Could you check a few things on this model? Use its own coordinates, in mm. Face numbers are marked on the shaded views. A direction names the side the tool comes from. Coordinates: 2 decimals unless noted, no trailing zeros. Loops run counter-clockwise (first coordinate to the right, second up) from the corner with the lowest first, then second, coordinate; pieces in that order, holes last.
1) Imagine slicing it at B-B on x = -8. Please give me the cut outline in (y, z), plus the area to 3 significant figures.
2) For the marked faces 1, 2, 3, 4 and 5, which set-ups out of +Z, -Z, +X, -X, +Y, -Y let a thin tool reach every point of the face, with its end or its side?
3) Imagine slicing it at A-A on z = 24.25. Please give me the cut outline in (x, y).
4) If I drill on line 1 along Z through (x, y) = (-0.25, 13); line 2 along X through (y, z) = (12, -12); line 3 along X through (y, z) = (3.5, -3), over which ranges is the centre line in solid material (lowest first)?
5) Imagine slicing it at D-D on x = 10.25. Please give me the cut outline in (y, z).
6) Imagine slicing it at C-C on y = 19.5. Please give me the cut outline in (x, z).
7) Will these pins go through, and if not, where does the flat tip stop? P1, Ø12, axis at x = -7, z = 8, coming from the +Y side; P2, Ø4, axis at x = 8, z = -12.25, coming from the -Y side; P3, Ø6.5, axis at x = -1.5, z = 12, coming from the -Y side.
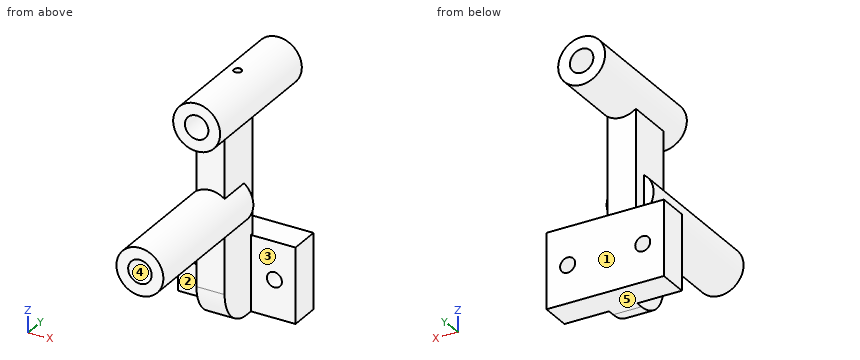
Autodesk Inventor part; units mm, degrees
ref_plane "Work Plane1" through (0, 0, 29.25) normal (0, 0, 1) x (1, 0, 0)
ref_plane "YZ Plane" through (0, 0, 0) normal (1, 0, 0) x (0, 1, 0)
ref_plane "XZ Plane" through (0, 0, 0) normal (0, 1, 0) x (-1, 0, 0)
sketch "Sketch1" plane through (0, 0, 0) normal (0, 1, 0) x (-1, 0, 0)
  line L0 (3, 20.25) -> (-3, 20.25)
  line L1 (-3, 20.25) -> (-3, -20.25)
  line L2 (-3, -20.25) -> (3, -20.25)
  line L3 (3, -20.25) -> (3, 20.25)
  line L4 (3, 20.25) -> (-3, -20.25) construction
  line L5 (-3, 20.25) -> (3, -20.25) construction
  point P0 (0, 0)
  dimension "d0" = 6
  dimension "d1" = 40.5
extrude "Extrusion1" add sketch "Sketch1" along normal blind 10
fillet "Fillet1" radius 8 1 edges at (0, 0, -20.25)
sketch "Sketch2" plane through (0, 10, 0) normal (0, 1, 0) x (1, 0, 0)
  line L0 (3, 20.25) -> (-3, 20.25) construction
  line L1 (0, 20.25) -> (0, -24.25) construction
  circle A0 centre (0, -24.25) radius 5
  point P0 (0, 0)
  dimension "d5" = 44.5
  dimension "d6" = 10
extrude "Extrusion2" add sketch "Sketch2" along normal blind 14.5 and the other way blind 15
sketch "Sketch3" plane through (0, 0, 0) normal (0, -1, 0) x (1, 0, 0)
  line L0 (3, -20.25) -> (-3, -20.25) construction
  line L1 (0, -20.25) -> (0, 3.75) construction
  circle A0 centre (0, 3.75) radius 5
  point P0 (0, 0)
  dimension "d11" = 24
  dimension "d12" = 10
extrude "Extrusion3" add sketch "Sketch3" along normal blind 25.5 and the other way blind 7
sketch "Sketch4" plane through (0, 10, 0) normal (0, 1, 0) x (1, 0, 0)
  line L0 (-3, 20.25) -> (3, 20.25) construction
  line L1 (0, 20.25) -> (0, 12.25) construction
  line L2 (-12.5, 4.25) -> (12.5, 4.25)
  line L3 (12.5, 4.25) -> (12.5, 20.25)
  line L4 (12.5, 20.25) -> (-12.5, 20.25)
  line L5 (-12.5, 20.25) -> (-12.5, 4.25)
  line L6 (-12.5, 4.25) -> (12.5, 20.25) construction
  line L7 (12.5, 4.25) -> (-12.5, 20.25) construction
  point P0 (0, 0)
  dimension "d17" = 8
  dimension "d18" = 25
extrude "Extrusion4" add sketch "Sketch4" along normal blind 6 and the other way blind 0.5
sketch "Sketch5" plane through (0, 16, 0) normal (0, 1, 0) x (1, 0, 0)
  line L0 (-3, 20.25) -> (3, 20.25) construction
  line L1 (0, 20.25) -> (0, 12.25) construction
  line L2 (0, 12.25) -> (-8, 12.25) construction
  circle A0 centre (-8, 12.25) radius 1.6
  circle A1 centre (8, 12.25) radius 1.6
  point P0 (0, 0)
  dimension "d23" = 8
  dimension "d24" = 8
  dimension "d25" = 3.2
extrude "Extrusion5" cut sketch "Sketch5" against normal through all
sketch "Sketch6" plane through (0, 24.5, 24.25) normal (0, 1, 0) x (1, 0, 0)
  circle A0 centre (0, 0) radius 2.5
  point P0 (0, 24.25)
  dimension "d28" = 5
extrude "Extrusion6" cut sketch "Sketch6" against normal through all
sketch "Sketch7" plane through (0, -25.5, 3.75) normal (0, -1, 0) x (1, 0, 0)
  circle A0 centre (0, 0) radius 1.3196
  point P0 (0, -3.75)
hole "Hole1" at (0, -25.5, 3.75) direction (0, 1, 0) diameter 5 depth 13 tip angle 118
ref_plane "Work Plane1" through (0, 0, 29.25) normal (0, 0, 1) x (1, 0, 0)
sketch "Sketch8" plane through (0, 0, 29.25) normal (0, 0, 1) x (1, 0, 0)
  line L0 (5, 24.5) -> (-5, 24.5)
  line L1 (0, 24.5) -> (0, 9.75)
  circle A0 centre (0, 9.75) radius 0.8
  point P0 (0, 0)
  dimension "d39" = 14.75
  dimension "d40" = 1.6
hole "Hole2" at (0, 9.75, 29.25) direction (0, 0, -1) diameter 1.6 end up to surface countersink diameter 1.7 countersink angle 45
properties part number "Supporto DX"
Filled in:
1. outline: (9.5, -20.25) - (16, -20.25) - (16, -13.85) - (9.5, -13.85) - close; (9.5, -10.65) - (16, -10.65) - (16, -4.25) - (9.5, -4.25) - close
1. area: 83.2 mm2
2. face 1: -Z, +X, -X, +Y
2. face 2: -Z, -X, -Y
2. face 3: -Z, +X, -Y
2. face 4: -Y
2. face 5: -Z, +X, -X, +Y, -Y
3. outline: (-5, -5) - (-2.5, -5) - (-2.5, 24.5) - (-5, 24.5) - close; (2.5, -5) - (5, -5) - (5, 24.5) - (2.5, 24.5) - close
4. line 1: z = -20.25 to -4.25, 19.26 to 21.76, 26.74 to 29.24
4. line 2: x = -12.5 to -9.58, -6.42 to 6.42, 9.58 to 12.5
4. line 3: x = -3 to 3
5. outline: (9.5, -20.25) - (16, -20.25) - (16, -4.25) - (9.5, -4.25) - close
6. outline: circle Ø10 at (0, 24.25); hole circle Ø5 at (0, 24.25)
7. P1: stops at y = 10
7. P2: stops at y = 9.5
7. P3: stops at y = 0
